The model under review builds one solid part; all positions refer to its coordinate system, in mm. Give positions to 0.01 mm unless a question says otherwise; leave off trailing zeros. Loops run counter-clockwise (first coordinate to the right, second up) from the corner with the lowest first, then second, coordinate; pieces in that order, holes last. Notation, with made-up numbers: M 19,-31 L 63,-31 A20 cw 63,-24 Z; hole C 44,4 d3. An arc over 180 degrees is marked long. Return JSON: item names as keys, results as strings.
```python
from build123d import *

# Parameters (mm, degrees)
SKETCH1_W               = 180
SKETCH1_H               = 100
BOSS_EXTRUDE1_DEPTH     = 5
SKETCH2_W               = 177
SKETCH2_H               = 97
BOSS_EXTRUDE2_DEPTH     = 1.5
CUT_EXTRUDE1_REACH      = 120.309
SKETCH3_W               = 61.468
SKETCH3_H               = 56.896
FILLET3_R               = 4
FILLET4_R               = 4
SKETCH5_W               = 2
SKETCH5_H               = 11
BOSS_EXTRUDE3_DEPTH     = 55
SKETCH7_W               = 2
SKETCH7_H               = 11
BOSS_EXTRUDE4_DEPTH     = 55
CUT_EXTRUDE3_DEPTH      = 153.194061156
CUT_EXTRUDE3_DEPTH_BACK = 153.194061156


with BuildPart() as part:
    # Sketch1 → Boss-Extrude1 (new body)
    with BuildSketch(Plane(origin=(0, 0, 0), x_dir=(1, 0, 0), z_dir=(0, 1, 0))):
        with Locations((11.492537313, -10.447761194)):
            Rectangle(SKETCH1_W, SKETCH1_H)
    extrude(amount=BOSS_EXTRUDE1_DEPTH)

    # Sketch2 → Boss-Extrude2 (add)
    with BuildSketch(Plane(origin=(0, 5, 0), x_dir=(1, 0, 0), z_dir=(0, 1, 0))):
        with Locations((11.492537313, -10.447761194)):
            Rectangle(SKETCH2_W, SKETCH2_H)
    extrude(amount=BOSS_EXTRUDE2_DEPTH)

    # Sketch3 → Cut-Extrude1 (cut, up to next)
    with BuildSketch(Plane(origin=(0, 6.5, 0), x_dir=(1, 0, 0), z_dir=(0, 1, 0)), mode=Mode.PRIVATE) as cut_extrude1_sk1:
        with Locations((63.60476585, 4.678190655)):
            Rectangle(SKETCH3_W, SKETCH3_H)
    cut_extrude1_tool1 = extrude(cut_extrude1_sk1.sketch, amount=-CUT_EXTRUDE1_REACH, mode=Mode.PRIVATE) & part.part
    add(cut_extrude1_tool1.solids().sort_by_distance((63.604766, 6.5, -4.678191))[0], mode=Mode.SUBTRACT)

    # Fillet3
    fillet3_edges = [part.edges().sort_by_distance(p)[0] for p in [
        (-78.507462687, 2.5, -39.552238806),
        (101.492537313, 2.5, -39.552238806),
        (101.492537313, 2.5, 60.447761194),
        (-78.507462687, 2.5, 60.447761194),
    ]]
    fillet(fillet3_edges, radius=FILLET3_R)

    # Fillet4
    fillet4_edges = [part.edges().sort_by_distance(p)[0] for p in [
        (11.492537313, 0, 60.447761194),
        (-78.507462687, 0, 10.447761194),
        (11.492537313, 0, -39.552238806),
        (101.492537313, 0, 10.447761194),
        (100.320964438, 0, 59.276188319),
        (100.320964438, 0, -38.380665931),
        (-77.335889811, 0, -38.380665931),
        (-77.335889811, 0, 59.276188319),
    ]]
    fillet(fillet4_edges, radius=FILLET4_R)

    # Sketch5 → Boss-Extrude3 (add)
    with BuildSketch(Plane(origin=(0, 6.5, 0), x_dir=(1, 0, 0), z_dir=(0, 1, 0))):
        with Locations((-46.337817573, -31.927761194)):
            Rectangle(SKETCH5_W, SKETCH5_H)
    extrude(amount=BOSS_EXTRUDE3_DEPTH)

    # Sketch7 → Boss-Extrude4 (add)
    with BuildSketch(Plane(origin=(0, 6.5, 0), x_dir=(1, 0, 0), z_dir=(0, 1, 0))):
        with Locations((45.899277236, -31.927761194)):
            Rectangle(SKETCH7_W, SKETCH7_H)
    extrude(amount=BOSS_EXTRUDE4_DEPTH)

    # Sketch8 → Cut-Extrude3 (cut, two sides: drawn at the far end of the back side and taken through both)
    with BuildSketch(Plane(origin=(46.899277236, 0, 0), x_dir=(0, 0, -1), z_dir=(1, 0, 0)).offset(-CUT_EXTRUDE3_DEPTH_BACK)):
        Polygon((-37.427761194, 61.5), (-37.427761194, 6.5), (-26.427761194, 47.552558883), (-26.427761194, 61.5), align=None)
    extrude(amount=CUT_EXTRUDE3_DEPTH + CUT_EXTRUDE3_DEPTH_BACK, mode=Mode.SUBTRACT)


solid = part.part
```
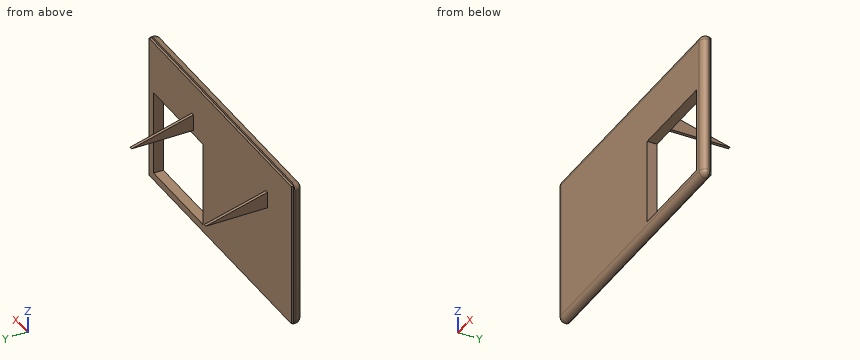
1) Insertion check: pin 1 (3 mm diameter, centred on y = 3, z = 9, fed in from +X); pin 2 (6 mm diameter, centred on x = -1, z = 44, fed in from +Y); pin 3 (1.6 mm diameter, centred on x = -46.5, y = 21.5, fed in from -Z); pin 4 (12 mm diameter, centred on y = 31, z = 30.5, fed in from -X). Each pin has a flat end and moves straight along its axis. Give the tip position at first contact, or say it passes through.
From the geometry:
{"pin 1": "x = 101.49", "pin 2": "y = 6.5", "pin 3": "z = 26.43", "pin 4": "x = -47.34"}
2) Consider section D-D on x = -60. Write out the cut boundary in (y, z).
From the geometry:
{"outline": "M 0,-35.55 A4 ccw 4,-39.55 L 5,-39.55 L 5,-38.05 L 6.5,-38.05 L 6.5,58.95 L 5,58.95 L 5,60.45 L 4,60.45 A4 ccw 0,56.45 Z"}
3) Wall thickness on L1, parallel to X at y = 9, z = 30.5; L2, parallel to Y at x = 4.5, z = -18; L3, parallel to Z at x = 91, y = 6: over which ranges is each line inside the solid? List them lowest first. Write a range as from..to.
From the geometry:
{"L1": "-47.34..-45.34, 44.9..46.9", "L2": "0..6.5", "L3": "-38.05..-33.13, 23.77..58.95"}
4) Consider section B-B on z = -9. Write out the cut boundary in (x, y).
From the geometry:
{"outline": "M -78.51,4 A4 ccw -74.51,0 L 32.87,0 L 32.87,6.5 L -77.01,6.5 L -77.01,5 L -78.51,5 Z; M 94.34,0 L 97.49,0 A4 ccw 101.49,4 L 101.49,5 L 99.99,5 L 99.99,6.5 L 94.34,6.5 Z"}
5) Consider section A-A on x = 41. Write out the cut boundary in (y, z).
From the geometry:
{"outline": "M 0,-35.55 A4 ccw 4,-39.55 L 5,-39.55 L 5,-38.05 L 6.5,-38.05 L 6.5,-33.13 L 0,-33.13 Z; M 0,23.77 L 6.5,23.77 L 6.5,58.95 L 5,58.95 L 5,60.45 L 4,60.45 A4 ccw 0,56.45 Z"}
6) Consider section C-C on y = 28. Write out the cut boundary in (x, z), then the cut area to 3 significant figures.
From the geometry:
{"outline": "M -47.34,26.43 L -45.34,26.43 L -45.34,31.67 L -47.34,31.67 Z; M 44.9,26.43 L 46.9,26.43 L 46.9,31.67 L 44.9,31.67 Z", "area": "21.0 mm²"}
